Can you work these out from the model? Positions are in its coordinate system, mm. A direction names the side the tool comes from. Give positions to 0.01 mm unless a question says otherwise; leave off trailing zeros. Write each loop counter-clockwise with the first axis right and the second up, starting at its lowest first coordinate (ties: lowest second). Pieces come first, ordered by that corner, then holes.
from build123d import *

# Parameters (mm, degrees)
BOSS_EXTRUDE1_DEPTH = 6
SKETCH3_W           = 5
SKETCH3_H           = 10
CUT_EXTRUDE2_DEPTH  = 10


with BuildPart() as part:
    # Sketch2 → Boss-Extrude1 (new body)
    with BuildSketch(Plane(origin=(0, 0, 0), x_dir=(1, 0, 0), z_dir=(0, 1, 0))):
        Polygon((121, 270), (121, 240.585), (115, 240.585), (115, 216.195), (121, 216.195), (121, 191.805), (115, 191.805), (115, 167.415), (121, 167.415), (121, 143.025), (121, 138), (133.805, 138), (133.805, 144), (158.195, 144), (158.195, 138), (171, 138), (171, 167.415), (177, 167.415), (177, 191.805), (171, 191.805), (171, 216.195), (177, 216.195), (177, 240.585), (171, 240.585), (171, 264.975), (171, 270), (158.195, 270), (158.195, 264), (133.805, 264), (133.805, 270), align=None)
    extrude(amount=BOSS_EXTRUDE1_DEPTH)

    # Sketch3 → Cut-Extrude2 (cut)
    with BuildSketch(Plane(origin=(0, 6, 0), x_dir=(1, 0, 0), z_dir=(0, 1, 0))):
        with Locations((168.5, 259)):
            Rectangle(SKETCH3_W, SKETCH3_H)
        with Locations((168.5, 223)):
            Rectangle(SKETCH3_W, SKETCH3_H)
        with Locations((168.5, 187)):
            Rectangle(SKETCH3_W, SKETCH3_H)
        with Locations((168.5, 151)):
            Rectangle(SKETCH3_W, SKETCH3_H)
    extrude(amount=-CUT_EXTRUDE2_DEPTH, mode=Mode.SUBTRACT)


solid = part.part
(1) For faces 3 (the face through (118, 3, -191.805)), 4 (the face through (168, 3, -182)), 5 (the face through (168, 3, -156)), 6 (the face through (133.805, 3, -267)), 7 (the face through (121, 3, -255)), which set-ups out of +Z, -Z, +X, -X, +Y, -Y let a thin tool reach every point of the face, with its end or its side?
Returned:
face 3: -X, +Y, -Y
face 4: +Y, -Y
face 5: +X, +Y, -Y
face 6: -Z, +Y, -Y
face 7: -Z, -X, +Y, -Y
(2) Imagine slicing it at B-B, the plane x = 153.5. Write out the boundary of the cut face in (y, z), plus the area to 3 significant figures.
Returned:
outline: (0, -264) - (6, -264) - (6, -144) - (0, -144) - close
area: 720 mm2
(3) If I drill on L1, parallel to X at y = 3.8, z = -226; L2, parallel to Z at x = 167.5, y = 5.15; L3, parallel to Z at x = 174, y = 4.35 (3 decimals), over which ranges is the centre line in solid material (lowest first)?
Returned:
L1: x = 115 to 166, 171 to 177
L2: z = -270 to -264, -254 to -228, -218 to -192, -182 to -156, -146 to -138
L3: z = -240.585 to -216.195, -191.805 to -167.415
(4) Imagine slicing it at A-A, the plane z = -189.5. Write out the boundary of the cut face in (x, y), plus the area to 3 significant figures.
Returned:
outline: (115, 0) - (166, 0) - (166, 6) - (115, 6) - close; (171, 0) - (177, 0) - (177, 6) - (171, 6) - close
area: 342 mm2
(5) Will these pins go through, and if not, where does the flat tip stop? P1, Ø1.8, axis at x = 175, y = 3, coming from the +Z side (3 decimals); P2, Ø2, axis at y = 4, z = -211.5, coming from the -X side; P3, Ø3, axis at y = 4, z = -266.5, coming from the +X side.
Returned:
P1: stops at z = -167.415
P2: stops at x = 121
P3: stops at x = 171
(6) If we mould it in two halves opening along Z, with no side actions, what happens to faces 1 (the face through (168, 3, -218)), 2 (the face through (146, 0, -205))? For each: +Z half, -Z half, draft (parallel to the pull), parting line (faces both ways), or undercut.
Returned:
face 1: undercut
face 2: draft
